Autodesk Inventor part; units mm, degrees
ref_plane "YZ Plane" through (0, 0, 0) normal (1, 0, 0) x (0, 1, 0)
ref_plane "XZ Plane" through (0, 0, 0) normal (0, 1, 0) x (-1, 0, 0)
ref_plane "XY Plane" through (0, 0, 0) normal (0, 0, 1) x (1, 0, 0)
sketch "Sketch1" plane through (0, 0, 0) normal (0, 0, 1) x (1, 0, 0)
  line L0 (-150, -75) -> (150, -75) construction
  line L1 (150, -75) -> (150, 75) construction
  line L2 (150, 75) -> (-150, 75) construction
  line L3 (-150, 75) -> (-150, -75) construction
  line L4 (-150, -75) -> (150, 75) construction
  line L5 (150, -75) -> (-150, 75) construction
  line L6 (147.5, -72.5) -> (-147.5, -72.5) construction
  line L7 (-147.5, -72.5) -> (-147.5, 72.5) construction
  line L8 (-147.5, 72.5) -> (147.5, 72.5) construction
  line L9 (147.5, 72.5) -> (147.5, -72.5) construction
  line L10 (147.5, -72.5) -> (-147.5, 72.5) construction
  line L11 (-147.5, -72.5) -> (147.5, 72.5) construction
  line L12 (-150, 75) -> (-146, 75) construction
  line L13 (-146, 75) -> (-146, 71) construction
  line L14 (-146, 71) -> (-150, 71) construction
  line L15 (-150, 71) -> (-150, 75) construction
  arc A0 (-146, 75) -> (-150, 71) centre (-146, 71) ccw
  line L16 (-150, -75) -> (-146, -75) construction
  line L17 (-146, -75) -> (-146, -71) construction
  line L18 (-146, -71) -> (-150, -71) construction
  line L19 (-150, -71) -> (-150, -75) construction
  line L20 (150, -75) -> (146, -75) construction
  line L21 (146, -75) -> (146, -71) construction
  line L22 (146, -71) -> (150, -71) construction
  line L23 (150, -71) -> (150, -75) construction
  line L24 (150, 75) -> (146, 75) construction
  line L25 (146, 75) -> (146, 71) construction
  line L26 (146, 71) -> (150, 71) construction
  line L27 (150, 71) -> (150, 75) construction
  line L28 (-146, 75) -> (146, 75)
  arc A1 (150, 71) -> (146, 75) centre (146, 71) ccw
  line L29 (150, 71) -> (150, -71)
  arc A2 (146, -75) -> (150, -71) centre (146, -71) ccw
  line L30 (146, -75) -> (-146, -75)
  arc A3 (-150, -71) -> (-146, -75) centre (-146, -71) ccw
  line L31 (-150, -71) -> (-150, 71)
  circle A4 centre (-146, 71) radius 2.5
  circle A5 centre (-146, -71) radius 2.5
  circle A6 centre (146, -71) radius 2.5
  circle A7 centre (146, 71) radius 2.5
  line L32 (-146, 71) -> (-142, 71) construction
  line L33 (-142, 71) -> (-142, 67) construction
  line L34 (-142, 67) -> (-146, 67) construction
  line L35 (-146, 67) -> (-146, 71) construction
  line L36 (-146, -71) -> (-142, -71) construction
  line L37 (-142, -71) -> (-142, -67) construction
  line L38 (-142, -67) -> (-146, -67) construction
  line L39 (-146, -67) -> (-146, -71) construction
  line L40 (146, -71) -> (142, -71) construction
  line L41 (142, -71) -> (142, -67) construction
  line L42 (142, -67) -> (146, -67) construction
  line L43 (146, -67) -> (146, -71) construction
  line L44 (146, 71) -> (142, 71) construction
  line L45 (142, 71) -> (142, 67) construction
  line L46 (142, 67) -> (146, 67) construction
  line L47 (146, 67) -> (146, 71) construction
  arc A8 (-146, 67) -> (-142, 71) centre (-146, 71) ccw
  arc A9 (-142, -71) -> (-146, -67) centre (-146, -71) ccw
  arc A10 (146, -67) -> (142, -71) centre (146, -71) ccw
  arc A11 (142, 71) -> (146, 67) centre (146, 71) ccw
  line L48 (-142, 71) -> (-140.5, 71) construction
  line L49 (-140.5, 71) -> (-140.5, 72.5) construction
  line L50 (-140.5, 72.5) -> (-142, 72.5) construction
  line L51 (-142, 72.5) -> (-142, 71) construction
  line L52 (-146, 67) -> (-147.5, 67) construction
  line L53 (-147.5, 67) -> (-147.5, 65.5) construction
  line L54 (-147.5, 65.5) -> (-146, 65.5) construction
  line L55 (-146, 65.5) -> (-146, 67) construction
  line L56 (142, 71) -> (140.5, 71) construction
  line L57 (140.5, 71) -> (140.5, 72.5) construction
  line L58 (140.5, 72.5) -> (142, 72.5) construction
  line L59 (142, 72.5) -> (142, 71) construction
  line L60 (146, 67) -> (147.5, 67) construction
  line L61 (147.5, 67) -> (147.5, 65.5) construction
  line L62 (147.5, 65.5) -> (146, 65.5) construction
  line L63 (146, 65.5) -> (146, 67) construction
  line L64 (146, -67) -> (147.5, -67) construction
  line L65 (147.5, -67) -> (147.5, -65.5) construction
  line L66 (147.5, -65.5) -> (146, -65.5) construction
  line L67 (146, -65.5) -> (146, -67) construction
  line L68 (142, -71) -> (140.5, -71) construction
  line L69 (140.5, -71) -> (140.5, -72.5) construction
  line L70 (140.5, -72.5) -> (142, -72.5) construction
  line L71 (142, -72.5) -> (142, -71) construction
  line L72 (-142, -71) -> (-140.5, -71) construction
  line L73 (-140.5, -71) -> (-140.5, -72.5) construction
  line L74 (-140.5, -72.5) -> (-142, -72.5) construction
  line L75 (-142, -72.5) -> (-142, -71) construction
  line L76 (-146, -67) -> (-147.5, -67) construction
  line L77 (-147.5, -67) -> (-147.5, -65.5) construction
  line L78 (-147.5, -65.5) -> (-146, -65.5) construction
  line L79 (-146, -65.5) -> (-146, -67) construction
  arc A12 (-147.5, -65.5) -> (-146, -67) centre (-146, -65.5) ccw
  arc A13 (-142, -71) -> (-140.5, -72.5) centre (-140.5, -71) ccw
  arc A14 (-140.5, 72.5) -> (-142, 71) centre (-140.5, 71) ccw
  arc A15 (-146, 67) -> (-147.5, 65.5) centre (-146, 65.5) ccw
  arc A16 (140.5, -72.5) -> (142, -71) centre (140.5, -71) ccw
  arc A17 (146, -67) -> (147.5, -65.5) centre (146, -65.5) ccw
  line L80 (147.5, -65.5) -> (147.5, 65.5)
  arc A18 (147.5, 65.5) -> (146, 67) centre (146, 65.5) ccw
  arc A19 (142, 71) -> (140.5, 72.5) centre (140.5, 71) ccw
  line L81 (140.5, 72.5) -> (-140.5, 72.5)
  line L82 (-147.5, 65.5) -> (-147.5, -65.5)
  line L83 (-140.5, -72.5) -> (140.5, -72.5)
  line L84 (146, 75) -> (-146, 75)
  arc A20 (-146, 75) -> (-150, 71) centre (-146, 71) ccw
  line L85 (-150, 71) -> (-150, -71)
  arc A21 (-150, -71) -> (-146, -75) centre (-146, -71) ccw
  line L86 (-146, -75) -> (146, -75)
  arc A22 (146, -75) -> (150, -71) centre (146, -71) ccw
  line L87 (150, -71) -> (150, 71)
  arc A23 (150, 71) -> (146, 75) centre (146, 71) ccw
  arc A24 (142, 71) -> (146, 67) centre (146, 71) ccw
  arc A25 (142, 71) -> (140.5, 72.5) centre (140.5, 71) ccw
  line L88 (140.5, 72.5) -> (-140.5, 72.5)
  arc A26 (-140.5, 72.5) -> (-142, 71) centre (-140.5, 71) ccw
  arc A27 (-146, 67) -> (-142, 71) centre (-146, 71) ccw
  arc A28 (-146, 67) -> (-147.5, 65.5) centre (-146, 65.5) ccw
  line L89 (-147.5, 65.5) -> (-147.5, -65.5)
  arc A29 (-147.5, -65.5) -> (-146, -67) centre (-146, -65.5) ccw
  arc A30 (-142, -71) -> (-146, -67) centre (-146, -71) ccw
  arc A31 (-142, -71) -> (-140.5, -72.5) centre (-140.5, -71) ccw
  line L90 (-140.5, -72.5) -> (140.5, -72.5)
  arc A32 (140.5, -72.5) -> (142, -71) centre (140.5, -71) ccw
  arc A33 (146, -67) -> (142, -71) centre (146, -71) ccw
  arc A34 (146, -67) -> (147.5, -65.5) centre (146, -65.5) ccw
  line L91 (147.5, -65.5) -> (147.5, 65.5)
  arc A35 (147.5, 65.5) -> (146, 67) centre (146, 65.5) ccw
  point P0 (0, 0)
  dimension "d0" = 300
  dimension "d1" = 150
  dimension "d2" = 295
  dimension "d3" = 145
  dimension "d4" = 4
  dimension "d5" = 4
  dimension "d6" = 4
  dimension "d7" = 4
  dimension "d8" = 4
  dimension "d9" = 4
  dimension "d10" = 4
  dimension "d11" = 4
  dimension "d12" = 4
  dimension "d13" = 4
  dimension "d14" = 4
  dimension "d15" = 4
  dimension "d16" = 5
  dimension "d17" = 5
  dimension "d18" = 5
  dimension "d19" = 5
  dimension "d20" = 4
  dimension "d21" = 4
  dimension "d22" = 4
  dimension "d23" = 4
  dimension "d24" = 4
  dimension "d25" = 4
  dimension "d26" = 4
  dimension "d27" = 4
  dimension "d28" = 4
  dimension "d29" = 4
  dimension "d30" = 4
  dimension "d31" = 4
  dimension "d32" = 1.5
  dimension "d33" = 1.5
  dimension "d34" = 1.5
  dimension "d35" = 1.5
  dimension "d36" = 1.5
  dimension "d37" = 1.5
  dimension "d38" = 1.5
  dimension "d39" = 1.5
  dimension "d40" = 1.5
  dimension "d41" = 1.5
  dimension "d42" = 1.5
  dimension "d43" = 1.5
  dimension "d44" = 1.5
  dimension "d45" = 1.5
  dimension "d46" = 1.5
  dimension "d47" = 1.5
  dimension "d48" = 1.5
  dimension "d49" = 1.5
  dimension "d50" = 1.5
  dimension "d51" = 1.5
  dimension "d52" = 1.5
  dimension "d53" = 1.5
  dimension "d54" = 1.5
  dimension "d55" = 1.5
extrude "Extrusion1" add sketch "Sketch1" along normal blind 2.5 contours L28 A1 L29 A2 L30 A3 L31 A0 | A8 A14 L81 A19 A11 A18 L80 A17 A10 A16 L83 A13 A9 A12 L82 A15
extrude "Extrusion2" add sketch "Sketch1" along normal blind 37.5
extrude "Extrusion3" add sketch "Sketch1" along normal blind 35.5 contours A4 | A5 | A6 | A7
equation "\"d21\" = d20"
properties part number "electronics_box"
Geometry check sheet. Reference: the model listing, model coordinates, mm. A direction names the side the tool comes from. Coordinates: 2 decimals unless noted, no trailing zeros. Order: outer loops, then holes, each group sorted by start corner. A loop starts at its lowest first (then second) coordinate and runs counter-clockwise, first axis right, second up.
Item 1: Mould release check, pull along X, two halves, no side actions. Record for faces 1 (the flat face through (150, 1, 18)), 2 (the flat face through (-2, 1, 2.5)), 3 (the flat face through (-2, 1, 0)): released by +X, released by -X, zero draft, split by the parting line, or undercut.
Item 2: Tool access check on faces 4 (the flat face through (-150, -1, 18)), 5 (the flat face through (147.5, -1, 20)). Record the directions out of +Z, -Z, +X, -X, +Y, -Y that give a thin tool (end or side, any length) a straight path to the whole face; none if there is none.
Item 3: Scan lines: line 1 along Y through (x, z) = (146, 36.4); line 2 along Y through (x, z) = (-120.5, 23); line 3 along X through (y, z) = (-14.5, 14). Record each from-to range of solid material in increasing order.
Item 4: Section check C-C (x = 121.5). Enter the section's corners in (y, z).
Item 5: Depth check by flat-ended pin: pin 1 (3 mm diameter, centred on x = -146, y = 71, fed in from +Z); pin 2 (2 mm diameter, centred on x = -82.5, y = -45.5, fed in from +Z). Enter the tip coordinate at first touch or a pass-through.
Item 6: Section check B-B (y = 16). Enter the section's corners in (x, z).
Item 7: Section check A-A (z = 21.5). Enter the section's corners in (x, y), plus the area to 3 significant figures.
Check sheet entries:
1. face 1: released by +X
1. face 2: undercut
1. face 3: zero draft
2. face 4: +Z, -Z, -X, +Y, -Y
2. face 5: +Z
3. line 1: y = -75 to -73.5, -68.5 to -67, 67 to 68.5, 73.5 to 75
3. line 2: y = -75 to -72.5, 72.5 to 75
3. line 3: x = -150 to -147.5, 147.5 to 150
4. outline: (-75, 0) - (75, 0) - (75, 37.5) - (72.5, 37.5) - (72.5, 2.5) - (-72.5, 2.5) - (-72.5, 37.5) - (-75, 37.5) - close
5. pin 1: stops at z = 35.5
5. pin 2: stops at z = 2.5
6. outline: (-150, 0) - (150, 0) - (150, 37.5) - (147.5, 37.5) - (147.5, 2.5) - (-147.5, 2.5) - (-147.5, 37.5) - (-150, 37.5) - close
7. outline: (-150, -71) arc R4 ccw to (-146, -75) - (146, -75) arc R4 ccw to (150, -71) - (150, 71) arc R4 ccw to (146, 75) - (-146, 75) arc R4 ccw to (-150, 71) - close; hole (-147.5, -65.5) arc R1.5 ccw to (-146, -67) arc R4 cw to (-142, -71) arc R1.5 ccw to (-140.5, -72.5) - (140.5, -72.5) arc R1.5 ccw to (142, -71) arc R4 cw to (146, -67) arc R1.5 ccw to (147.5, -65.5) - (147.5, 65.5) arc R1.5 ccw to (146, 67) arc R4 cw to (142, 71) arc R1.5 ccw to (140.5, 72.5) - (-140.5, 72.5) arc R1.5 ccw to (-142, 71) arc R4 cw to (-146, 67) arc R1.5 ccw to (-147.5, 65.5) - close
7. area: 2,320 mm2
